Geometry: final body of the model. Coordinates: model frame, mm. Give positions to 0.01 mm unless a question says otherwise; leave off trailing zeros. Write each loop counter-clockwise with the first axis right and the second up, starting at its lowest first coordinate (ties: lowest second). Pieces come first, ordered by that corner, then holes. Notation, with made-up numbers: (43.25, 66.25) - (83.25, 66.25) arc R22 cw to (83.25, 95.25) - close; hole circle Ø8 at (81.5, 9). An arc over 180 degrees is marked (long way). Return JSON: item names as keys, results as strings.
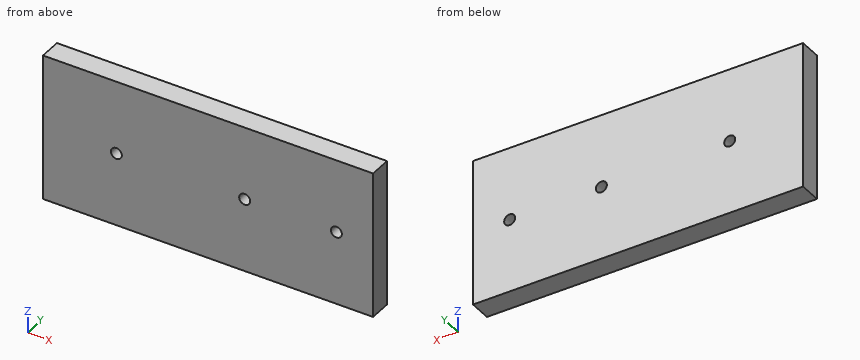
from build123d import *

# Parameters (mm, degrees)
F0_W     = 90
F0_H     = 40
F0_R     = 1.5
F1_DEPTH = 3


with BuildPart() as f1:
    # F0 (on Front) → F1 (new body, symmetric)
    with BuildSketch(Plane.XZ):
        with Locations((-45, 20)):
            Rectangle(F0_W, F0_H)
        with Locations((-70, 20)):
            Circle(F0_R, mode=Mode.SUBTRACT)
        with Locations((-35, 20)):
            Circle(F0_R, mode=Mode.SUBTRACT)
        with Locations((-10, 20)):
            Circle(F0_R, mode=Mode.SUBTRACT)
    extrude(amount=F1_DEPTH, both=True)


solid = f1.part
Q1. Pin query (flat end, axial travel): P1, Ø1.5, axis at y = 1, z = 25, coming from the +X side. Return the tip coordinate at first contact, or that it passes through.
Answer key:
{"P1": "stops at x = 0"}
Q2. Material intervals for probe 1 along Z at (x, y) = (-35, -0.45), sorted ascending. Write a range as [from, to].
Answer key:
{"probe 1": "z = [0, 18.5], [21.5, 40]"}
Q3. Section query B-B, the plane x = -70. Return the cut outline in (y, z), plus the area to 3 significant figures.
Answer key:
{"outline": "(-3, 0) - (3, 0) - (3, 18.5) - (-3, 18.5) - close; (-3, 21.5) - (3, 21.5) - (3, 40) - (-3, 40) - close", "area": "222 mm^2"}
Q4. Section query A-A, the plane z = 20. Return the cut outline in (x, y), plus the area to 3 significant figures.
Answer key:
{"outline": "(-90, -3) - (-71.5, -3) - (-71.5, 3) - (-90, 3) - close; (-68.5, -3) - (-36.5, -3) - (-36.5, 3) - (-68.5, 3) - close; (-33.5, -3) - (-11.5, -3) - (-11.5, 3) - (-33.5, 3) - close; (-8.5, -3) - (0, -3) - (0, 3) - (-8.5, 3) - close", "area": "486 mm^2"}
